```python
from build123d import *

# Parameters (mm, degrees)
CYLINDER002_R     = 38.4
CYLINDER002_DEPTH = 1
CYLINDER001_R     = 48.4
CYLINDER001_DEPTH = 1


with BuildPart() as bottom_wall_cutout:
    # Cylinder002 → Cylinder002 (new body)
    with BuildSketch(Plane.XY.offset(-1)):
        Circle(CYLINDER002_R)
    extrude(amount=CYLINDER002_DEPTH)


with BuildPart() as bottom_flange:
    # Cylinder001 → Cylinder001 (new body)
    with BuildSketch(Plane.XY.offset(-1)):
        Circle(CYLINDER001_R)
    extrude(amount=CYLINDER001_DEPTH)

    # Cut002: cut bottom_wall_cutout
    add(bottom_wall_cutout.part, mode=Mode.SUBTRACT)


solid = bottom_flange.part
```
Input: part model. Units: mm. Frame: model coordinates. Give positions to 0.01 mm unless a question says otherwise; leave off trailing zeros. Order: outer loops, then holes, each group sorted by start corner. A loop starts at its lowest first (then second) coordinate and runs counter-clockwise, first axis right, second up.
1. Section A-A on y = 0. Return the cut outline in (x, z), and give its area (3 significant figures).
Derived:
outline: (-48.4, -1) - (-38.4, -1) - (-38.4, 0) - (-48.4, 0) - close; (38.4, -1) - (48.4, -1) - (48.4, 0) - (38.4, 0) - close
area: 20.0 mm2
2. Material intervals for L1, parallel to Y at x = 0, z = -0.8; L2, parallel to Y at x = -3.5, z = -0.3; L3, parallel to X at y = -12.5, z = -0.4, sorted ascending.
Derived:
L1: y = -48.4 to -38.4, 38.4 to 48.4
L2: y = -48.27 to -38.24, 38.24 to 48.27
L3: x = -46.76 to -36.31, 36.31 to 46.76
3. Mould query, pull axis Y, two halves, no side actions, for faces 1 (the cylindrical face through (20.64, 32.38, -0.51)), 2 (the flat face through (-15, 36, 0)), 3 (the cylindrical face through (44.71, -18.54, -0.51)). Classes: released by +Y, released by -Y, zero draft, split by the parting line, or undercut.
Derived:
face 1: undercut
face 2: zero draft
face 3: split by the parting line
4. Section C-C on z = -0.5. Return the cut outline in (x, y).
Derived:
outline: circle Ø96.8 at (0, 0); hole circle Ø76.8 at (0, 0)
5. Section D-D on x = -41. Return the cut outline in (y, z).
Derived:
outline: (-25.72, -1) - (25.72, -1) - (25.72, 0) - (-25.72, 0) - close
